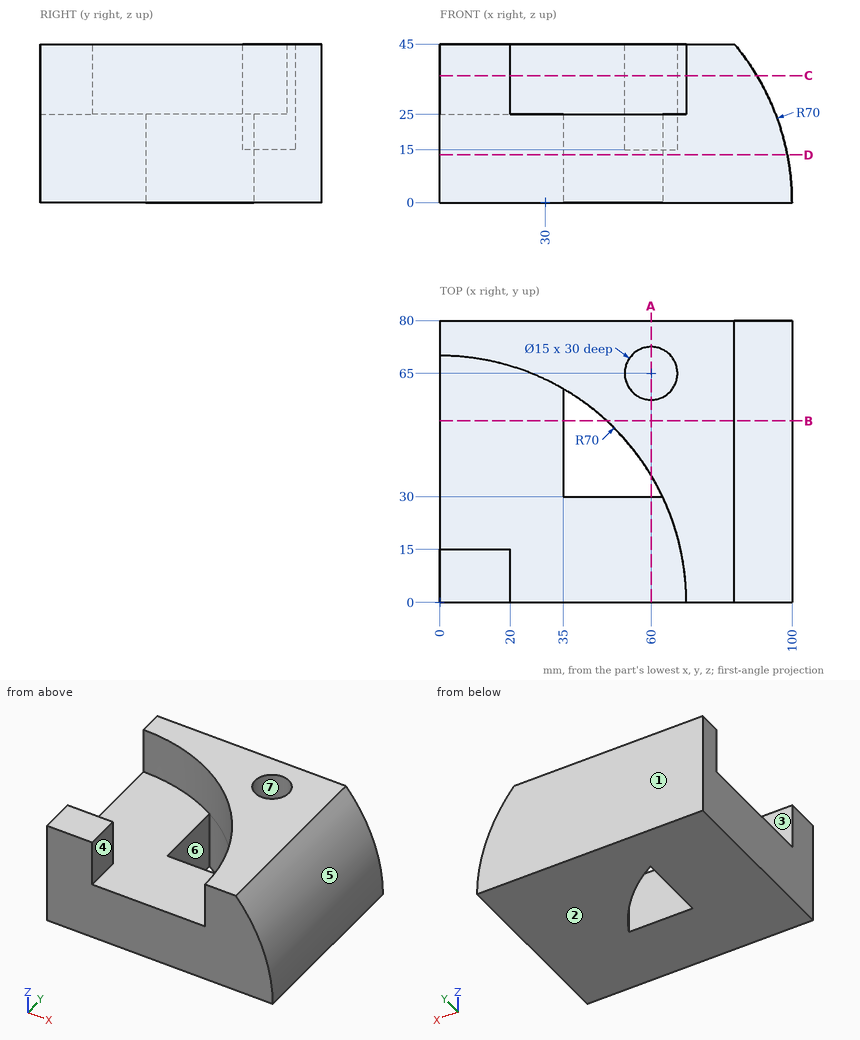
Job drawing, mm, ordinate dimensions from the low corner. One solid piece. A direction names the side the tool comes from. Give positions to 0.01 mm unless a question says otherwise; leave off trailing zeros. Loops run counter-clockwise (first coordinate to the right, second up) from the corner with the lowest first, then second, coordinate; pieces in that order, holes last. Notation, with made-up numbers: (53.5, 35.5) - (90.5, 35.5) arc R20 ccw to (90.5, 42.5) - close; hole circle Ø2 at (-26, 23). An arc over 180 degrees is marked (long way). Use one line per item in the form item = value.
(1) Cut at B-B (y = 51.5). Give the cut face in (x, z).
Determined:
outline = (0, 0) - (35, 0) - (35, 25) - (0, 25) - close; (47.41, 0) - (100, 0) arc R70 ccw to (83.62, 45) - (47.41, 45) - close
(2) Cut at D-D (z = 13.5). Give the cut face in (x, y).
Determined:
outline = (0, 0) - (98.69, 0) - (98.69, 80) - (0, 80) - close; hole (35, 30) - (63.25, 30) arc R70 ccw to (35, 60.62) - close
(3) Cut at C-C (z = 36). Give the cut face in (x, y), then the cut area to 3 significant figures.
Determined:
outline = (0, 0) - (20, 0) - (20, 15) - (0, 15) - close; (0, 70) arc R70 cw to (70, 0) - (90.03, 0) - (90.03, 80) - (0, 80) - close; hole circle Ø15 at (60, 65)
area = 3,480 mm^2
(4) 3-axis set-ups, long thin cutter, end or side, ignore diameter. For the marked faces 4, 5, 6 and 7: which of +Z, -Z, +X, -X, +Y, -Y reach the whole face in a straight line?
Determined:
face_4 = +Z, -Y
face_5 = +Z, +X, +Y, -Y
face_6 = +Z, -Z
face_7 = +Z
(5) Drill centre lines: L1, parallel to Y at x = 60, z = 23; L2, parallel to Z at x = 22.5, y = 5; L3, parallel to Y at x = 60, z = 27.25. Where is each one in solid material? Low to high.
Determined:
L1 = 0 to 30, 36.06 to 57.5, 72.5 to 80
L2 = 0 to 25
L3 = 36.06 to 57.5, 72.5 to 80
(6) Drop flat-ended pins along their axis: P1, Ø3, axis at y = 22.5, z = 36, coming from the +X side; P2, Ø3, axis at y = 20.5, z = 27, coming from the -X side; P3, Ø4.5, axis at x = 59.5, y = 63.5, coming from the +Z side. Give the stop position or say it passes through.
Determined:
P1 = 90.91
P2 = 66.45
P3 = 15
(7) Pull direction Y, two halves, no side cores. Call the marked faces 1, 2 and 3: pulls with the +Y half, pulls with the -Y half, needs draft (parallel to the pull), parting line crosses it, or undercut.
Determined:
face_1 = pulls with the +Y half
face_2 = needs draft
face_3 = undercut
(8) Cut at A-A (x = 60). Give the cut face in (y, z).
Determined:
outline = (0, 0) - (30, 0) - (30, 25) - (0, 25) - close; (36.06, 0) - (80, 0) - (80, 45) - (72.5, 45) - (72.5, 15) - (57.5, 15) - (57.5, 45) - (36.06, 45) - close
